Build history of the part. All positions in model axes, mm. A direction names the side the tool comes from. Give positions to 0.01 mm unless a question says otherwise; leave off trailing zeros. Write each loop counter-clockwise with the first axis right and the second up, starting at its lowest first coordinate (ties: lowest second). Pieces come first, ordered by that corner, then holes. Notation, with made-up numbers: (81, 87.25) -> (108, 87.25) arc R29 cw to (108, 116.25) -> close; hole circle Ø5 at (-32, -26.75). An arc over 180 degrees is marked (long way). Put each result on its own line as item: value.
from build123d import *

# Parameters (mm, degrees)
SKETCH2_W           = 60
SKETCH2_H           = 60
BOSS_EXTRUDE1_DEPTH = 15
SKETCH3_R           = 5.05
CUT_EXTRUDE3_DEPTH  = 3
SKETCH5_R           = 3.1
CUT_EXTRUDE4_DEPTH  = 12
SKETCH6_R           = 2.75
CUT_EXTRUDE5_DEPTH  = 5.5


with BuildPart() as part:
    # Sketch2 → Boss-Extrude1 (new body)
    with BuildSketch(Plane(origin=(0, 0, 0), x_dir=(1, 0, 0), z_dir=(0, 1, 0))):
        Rectangle(SKETCH2_W, SKETCH2_H)
    extrude(amount=BOSS_EXTRUDE1_DEPTH)

    # Sketch3 → Cut-Extrude3 (cut)
    with BuildSketch(Plane(origin=(0, 15, 0), x_dir=(1, 0, 0), z_dir=(0, 1, 0))):
        with Locations(Location((-21.804493365, 0, 0), (0, 0, 270))):
            Circle(SKETCH3_R)
    extrude(amount=-CUT_EXTRUDE3_DEPTH, mode=Mode.SUBTRACT)

    # Sketch5 → Cut-Extrude4 (cut)
    with BuildSketch(Plane(origin=(0, 0, 0), x_dir=(1, 0, 0), z_dir=(0, 1, 0))):
        with Locations(Location((-21.804493365, 0, 0), (0, 0, 270))):
            Circle(SKETCH5_R)
    extrude(amount=CUT_EXTRUDE4_DEPTH, mode=Mode.SUBTRACT)

    # Sketch6 → Cut-Extrude5 (cut)
    with BuildSketch(Plane(origin=(0, 15, 0), x_dir=(1, 0, 0), z_dir=(0, 1, 0))):
        with Locations(Location((20, 20, 0), (0, 0, 270))):
            Circle(SKETCH6_R)
    extrude(amount=-CUT_EXTRUDE5_DEPTH, mode=Mode.SUBTRACT)


solid = part.part
1) Wall check: L1, parallel to X at y = 1.5, z = 0; L2, parallel to X at y = 12.8, z = -20; L3, parallel to Y at x = 20, z = -18.5. Give the ranges that are in metal, low to high.
Filled sheet:
L1: -30 to -24.9, -18.7 to 30
L2: -30 to 17.25, 22.75 to 30
L3: 0 to 9.5
2) Slice it at C-C (x = 20). Write the cut outline in (y, z), plus the area to 3 significant figures.
Filled sheet:
outline: (0, -30) -> (15, -30) -> (15, -22.75) -> (9.5, -22.75) -> (9.5, -17.25) -> (15, -17.25) -> (15, 30) -> (0, 30) -> close
area: 870 mm2
3) Slice it at D-D (y = 13.5). Write the cut outline in (x, z).
Filled sheet:
outline: (-30, -30) -> (30, -30) -> (30, 30) -> (-30, 30) -> close; hole circle Ø10.1 at (-21.8, 0); hole circle Ø5.5 at (20, -20)
4) Tool access for faces 1 (the cylindrical face through (-16.797, 13.521, -0.657)), 2 (the flat face through (0, 7, -30)): list every direction of +Z, -Z, +X, -X, +Y, -Y with a clear straight run to the whole face (end or side of a thin tool).
Filled sheet:
face 1: +Y
face 2: -Z, +X, -X, +Y, -Y
5) Pull direction X, two halves, no side cores. Call faces 3 (the flat face through (0, 0, 0)), 4 (the flat face through (30, 7, 0)), 5 (the flat face through (-19, 12, 2)): released by +X, released by -X, zero draft, split by the parting line, or undercut.
Filled sheet:
face 3: zero draft
face 4: released by +X
face 5: undercut
6) Slice it at B-B (x = -21). Write the cut outline in (y, z).
Filled sheet:
outline: (0, -30) -> (15, -30) -> (15, -4.99) -> (12, -4.99) -> (12, -2.99) -> (0, -2.99) -> close; (0, 2.99) -> (12, 2.99) -> (12, 4.99) -> (15, 4.99) -> (15, 30) -> (0, 30) -> close
7) Slice it at A-A (z = 0). Write the cut outline in (x, y), plus the area to 3 significant figures.
Filled sheet:
outline: (-30, 0) -> (-24.9, 0) -> (-24.9, 12) -> (-26.85, 12) -> (-26.85, 15) -> (-30, 15) -> close; (-18.7, 0) -> (30, 0) -> (30, 15) -> (-16.75, 15) -> (-16.75, 12) -> (-18.7, 12) -> close
area: 795 mm2
